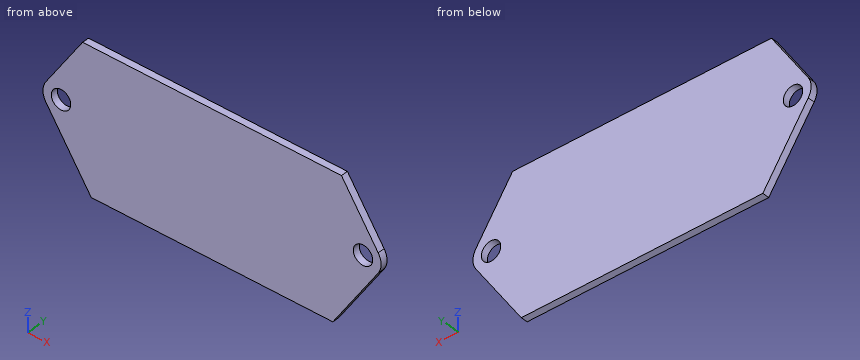
from build123d import *

# Parameters (mm, degrees)
SKETCH1_R           = 2.25
BOSS_EXTRUDE1_DEPTH = 1.6
FILLET1_R           = 4


with BuildPart() as part:
    # Sketch1 → Boss-Extrude1 (new body)
    with BuildSketch(Plane(origin=(0, 0, 0), x_dir=(1, 0, 0), z_dir=(0, 1, 0))):
        Polygon((12, 33), (0, 15), (10, 0), (70, 0), (80, 15), (68, 33), align=None)
        with Locations(Location((5, 15, 0), (0, 0, 270))):
            Circle(SKETCH1_R, mode=Mode.SUBTRACT)
        with Locations(Location((75, 15, 0), (0, 0, 270))):
            Circle(SKETCH1_R, mode=Mode.SUBTRACT)
    extrude(amount=BOSS_EXTRUDE1_DEPTH)

    # Fillet1
    fillet1_edges = [part.edges().sort_by_distance(p)[0] for p in [
        (0, 0.8, -15),
        (80, 0.8, -15),
    ]]
    fillet(fillet1_edges, radius=FILLET1_R)


solid = part.part
Check sheet for the modelled part. Datum: model origin and axes. Units: mm. Round coordinates to 2 decimals unless told otherwise and drop trailing zeros. Loops run counter-clockwise (first coordinate to the right, second up) from the corner with the lowest first, then second, coordinate; pieces in that order, holes last.
1. Sectioned sample at B-B on z = -15. Record the boundary of the cut face in (x, y), and give its area (3 significant figures).
2. Sectioned sample at D-D on z = -6.5. Record the boundary of the cut face in (x, y), and give its area (3 significant figures).
3. Sectioned sample at A-A on x = 5. Record the boundary of the cut face in (y, z).
4. Sectioned sample at C-C on y = 1.1. Record the boundary of the cut face in (x, z), and give its area (3 significant figures).
5. Scan lines: probe 1 along X at (y, z) = (0.7, -15); probe 2 along Z at (x, y) = (73, 0.5); probe 3 along X at (y, z) = (0.65, -4.5). Record each from-to range of solid material in increasing order.
Recorded:
1. outline: (0.81, 0) - (2.75, 0) - (2.75, 1.6) - (0.81, 1.6) - close; (7.25, 0) - (72.75, 0) - (72.75, 1.6) - (7.25, 1.6) - close; (77.25, 0) - (79.19, 0) - (79.19, 1.6) - (77.25, 1.6) - close
1. area: 111 mm2
2. outline: (5.67, 0) - (74.33, 0) - (74.33, 1.6) - (5.67, 1.6) - close
2. area: 110 mm2
3. outline: (0, -22.5) - (1.6, -22.5) - (1.6, -17.25) - (0, -17.25) - close; (0, -12.75) - (1.6, -12.75) - (1.6, -7.5) - (0, -7.5) - close
4. outline: (1.48, -17.22) - (12, -33) - (68, -33) - (78.52, -17.22) arc R4 ccw to (78.52, -12.78) - (70, 0) - (10, 0) - (1.48, -12.78) arc R4 ccw to start; hole circle Ø4.5 at (5, -15); hole circle Ø4.5 at (75, -15)
4. area: 2,240 mm2
5. probe 1: x = 0.81 to 2.75, 7.25 to 72.75, 77.25 to 79.19
5. probe 2: z = -25.5 to -16.03, -13.97 to -4.5
5. probe 3: x = 7 to 73
